Design review of the part built by this model. Coordinates are the model's own, in mm. Face numbers are marked on the shaded views. A direction names the side the tool comes from. Coordinates: 2 decimals unless noted, no trailing zeros. Loops run counter-clockwise (first coordinate to the right, second up) from the corner with the lowest first, then second, coordinate; pieces in that order, holes last.
Q1. Machinability: for the marked faces 4, 5 and 6, which of the approach directions +Z, -Z, +X, -X, +Y, -Y give a long, thin tool a straight path to every point of the face, cutting with its end or side? Answer none if there is none.
Q2. Wall thickness on probe 1 along Y at (x, z) = (0, 20); probe 2 along Y at (x, z) = (23.5, 9.5); probe 3 along Z at (x, y) = (8, 41): over which ranges is each line inside the solid? List them lowest first.
Q3. Add section A-A on x = 0. Give the boundary of the cut face in (y, z), and give its area (3 significant figures).
Q4. Add section C-C on x = -29.5. Give the boundary of the cut face in (y, z).
Q5. Draft analysis for pull direction X (two halves, no side actions). For the marked faces 1, 2 and 3, state which applies: released by +X, released by -X, zero draft, split by the parting line, or undercut.
Q6. Add section B-B on z = 30. Give the boundary of the cut face in (x, y).
Q7. For P1, Ø2, axis at x = -6.5, z = 31, coming from the -Y side; P2, Ø3, axis at x = 28.5, y = 12, coming from the +Z side; P3, Ø4, axis at x = -10.5, z = 16.5, coming from the +Y side; P4, Ø8, axis at y = 31, z = 22, coming from the +X side (3 decimals), all flat-tipped, find the tip position at first contact; note any pin that passes through.
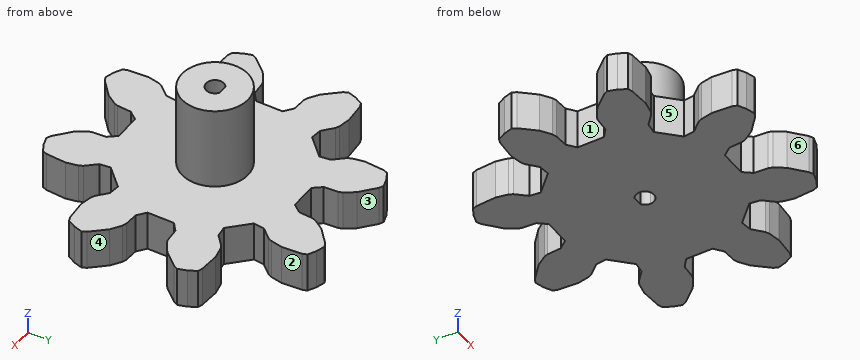
```python
from build123d import *

# Parameters (mm, degrees)
F1_DEPTH = 15.24
F2_R     = 12.7
F3_DEPTH = 31.75
F4_DEPTH = 25.4


with BuildPart() as f1:
    # F0 (on Top) → F1 (new body)
    with BuildSketch(Plane.XY):
        Polygon((-48.986719159, 25.3412460777), (-50.7255351294, 24.7465363945), (-52.3601977854, 21.688304154), (-53.366815822, 18.3699267661), (-52.5578082129, 16.719871907), (-47.6057296253, 11.0468524364), (-43.80914346, 8.4974130761), (-42.2801519731, 7.9744654227), (-37.0147232049, 7.6171909331), (-33.782, 5.0679251692), (-33.782, -5.0679251692), (-37.0147232049, -7.6171909331), (-42.2801519731, -7.9744654227), (-43.80914346, -8.4974130761), (-47.6057296253, -11.0468524364), (-52.5578082129, -16.719871907), (-53.366815822, -18.3699267661), (-52.3601977854, -21.688304154), (-50.7255351294, -24.7465363945), (-48.986719159, -25.3412460777), (-41.4736370284, -25.8510271212), (-36.9863201834, -24.9691669416), (-35.5353802528, -24.2577827562), (-31.559527, -20.7871925925), (-27.4710453735, -20.303918365), (-20.303918365, -27.4710453735), (-20.7871925925, -31.559527), (-24.2577827562, -35.5353802528), (-24.9691669416, -36.9863201834), (-25.8510271212, -41.4736370284), (-25.3412460777, -48.986719159), (-24.7465363945, -50.7255351294), (-21.688304154, -52.3601977854), (-18.3699267661, -53.366815822), (-16.719871907, -52.5578082129), (-11.0468524364, -47.6057296253), (-8.4974130761, -43.80914346), (-7.9744654227, -42.2801519731), (-7.6171909331, -37.0147232049), (-5.0679251692, -33.782), (5.0679251692, -33.782), (7.6171909331, -37.0147232049), (7.9744654227, -42.2801519731), (8.4974130761, -43.80914346), (11.0468524364, -47.6057296253), (16.719871907, -52.5578082129), (18.3699267661, -53.366815822), (21.688304154, -52.3601977854), (24.7465363945, -50.7255351294), (25.3412460777, -48.986719159), (25.8510271212, -41.4736370284), (24.9691669416, -36.9863201834), (24.2577827562, -35.5353802528), (20.7871925925, -31.559527), (20.303918365, -27.4710453735), (27.4710453735, -20.303918365), (31.559527, -20.7871925925), (35.5353802528, -24.2577827562), (36.9863201834, -24.9691669416), (41.4736370284, -25.8510271212), (48.986719159, -25.3412460777), (50.7255351294, -24.7465363945), (52.3601977854, -21.688304154), (53.366815822, -18.3699267661), (52.5578082129, -16.719871907), (47.6057296253, -11.0468524364), (43.80914346, -8.4974130761), (42.2801519731, -7.9744654227), (37.0147232049, -7.6171909331), (33.782, -5.0679251692), (33.782, 5.0679251692), (37.0147232049, 7.6171909331), (42.2801519731, 7.9744654227), (43.80914346, 8.4974130761), (47.6057296253, 11.0468524364), (52.5578082129, 16.719871907), (53.366815822, 18.3699267661), (52.3601977854, 21.688304154), (50.7255351294, 24.7465363945), (48.986719159, 25.3412460777), (41.4736370284, 25.8510271212), (36.9863201834, 24.9691669416), (35.5353802528, 24.2577827562), (31.559527, 20.7871925925), (27.4710453735, 20.303918365), (20.303918365, 27.4710453735), (20.7871925925, 31.559527), (24.2577827562, 35.5353802528), (24.9691669416, 36.9863201834), (25.8510271212, 41.4736370284), (25.3412460777, 48.986719159), (24.7465363945, 50.7255351294), (21.688304154, 52.3601977854), (18.3699267661, 53.366815822), (16.719871907, 52.5578082129), (11.0468524364, 47.6057296253), (8.4974130761, 43.80914346), (7.9744654227, 42.2801519731), (7.6171909331, 37.0147232049), (5.0679251692, 33.782), (-5.0679251692, 33.782), (-7.6171909331, 37.0147232049), (-7.9744654227, 42.2801519731), (-8.4974130761, 43.80914346), (-11.0468524364, 47.6057296253), (-16.719871907, 52.5578082129), (-18.3699267661, 53.366815822), (-21.688304154, 52.3601977854), (-24.7465363945, 50.7255351294), (-25.3412460777, 48.986719159), (-25.8510271212, 41.4736370284), (-24.9691669416, 36.9863201834), (-24.2577827562, 35.5353802528), (-20.7871925925, 31.559527), (-20.303918365, 27.4710453735), (-27.4710453735, 20.303918365), (-31.559527, 20.7871925925), (-35.5353802528, 24.2577827562), (-36.9863201834, 24.9691669416), (-41.4736370284, 25.8510271212), align=None)
        Polygon((-6.457554456, 6.1279886028), (-5.0423575535, 7.3366771559), (-3.4067913067, 8.2247200336), (-1.622328418, 8.7533028893), (0.2330374214, 8.8993240645), (2.0782189459, 8.6564005578), (3.8325695574, 8.0351529003), (5.4194220185, 7.0627288788), (6.7694179402, 5.7816284228), (7.8235568446, 4.247847459), (8.5357689507, 2.5284119549), (8.8749315621, 0.6984712932), (8.8262133252, -1.1619911548), (8.3917463583, -2.9716744665), (7.5905194232, -4.6514766054), (6.457554456, -6.1279886028), (5.0423575535, -7.3366771559), (3.4067913067, -8.2247200336), (1.622328418, -8.7533028893), (-0.2330374214, -8.8993240645), (-2.0782189459, -8.6564005578), (-3.8325695574, -8.0351529003), (-5.4194220185, -7.0627288788), (-6.7694179402, -5.7816284228), (-7.8235568446, -4.247847459), (-8.5357689507, -2.5284119549), (-8.8749315621, -0.6984712932), (-8.8262133252, 1.1619911548), (-8.3917463583, 2.9716744665), (-7.5905194232, 4.6514766054), align=None, mode=Mode.SUBTRACT)
        Polygon((-3.4067913067, 8.2247200336), (-5.0423575535, 7.3366771559), (-6.457554456, 6.1279886028), (-7.5905194232, 4.6514766054), (-8.3917463583, 2.9716744665), (-8.8262133252, 1.1619911548), (-8.8749315621, -0.6984712932), (-8.5357689507, -2.5284119549), (-7.8235568446, -4.247847459), (-6.7694179402, -5.7816284228), (-5.4194220185, -7.0627288788), (-3.8325695574, -8.0351529003), (-2.0782189459, -8.6564005578), (-0.2330374214, -8.8993240645), (1.622328418, -8.7533028893), (3.4067913067, -8.2247200336), (5.0423575535, -7.3366771559), (6.457554456, -6.1279886028), (7.5905194232, -4.6514766054), (8.3917463583, -2.9716744665), (8.8262133252, -1.1619911548), (8.8749315621, 0.6984712932), (8.5357689507, 2.5284119549), (7.8235568446, 4.247847459), (6.7694179402, 5.7816284228), (5.4194220185, 7.0627288788), (3.8325695574, 8.0351529003), (2.0782189459, 8.6564005578), (0.2330374214, 8.8993240645), (-1.622328418, 8.7533028893), align=None)
    extrude(amount=F1_DEPTH)

    # F2 (on face) → F3 (join)
    with BuildSketch(Plane.XY.offset(15.24)):
        Circle(F2_R)
        with BuildLine():
            ThreePointArc((1.7960512242, 2.921), (2.9930503377, 1.6732276223), (3.429, 0))
            ThreePointArc((3.429, 0), (-1.6732276223, -2.9930503377), (-1.7960512242, 2.921))
            ThreePointArc((-1.7960512242, 2.921), (0, 3.429), (1.7960512242, 2.921))
        make_face(mode=Mode.SUBTRACT)
        with BuildLine():
            Line((-1.7960512242, 2.921), (1.7960512242, 2.921))
            ThreePointArc((1.7960512242, 2.921), (0, 3.429), (-1.7960512242, 2.921))
        make_face()
    extrude(amount=F3_DEPTH)

    # F4 (cut): a face of the model
    f4_faces = [f1.faces().sort_by_distance(p)[0] for p in [
        (0, -0.108182678, 15.24),
    ]]
    extrude(f4_faces, amount=-F4_DEPTH, mode=Mode.SUBTRACT)


solid = f1.part
```
Entries:
1. face 4: +Z, -Z, +X
1. face 5: +Z, -Z
1. face 6: +Z, -Z, -Y
2. probe 1: y = -12.7 to -3.43, 2.92 to 12.7
2. probe 2: y = -51.39 to -34.67, -24.27 to 24.27, 34.67 to 51.39
2. probe 3: z = 0 to 15.24
3. outline: (-33.78, 0) - (-3.43, 0) - (-3.43, 46.99) - (-12.7, 46.99) - (-12.7, 15.24) - (-33.78, 15.24) - close; (2.92, 0) - (33.78, 0) - (33.78, 15.24) - (12.7, 15.24) - (12.7, 46.99) - (2.92, 46.99) - close
3. area: 1,540 mm2
4. outline: (-20.54, 0) - (20.54, 0) - (20.54, 15.24) - (-20.54, 15.24) - close
5. face 1: released by -X
5. face 2: released by +X
5. face 3: undercut
6. outline: circle Ø25.4 at (0, 0); hole (-1.8, 2.92) arc R3.43 ccw (long way) to (1.8, 2.92) - close
7. P1: stops at y = -11.45
7. P2: stops at z = 15.24
7. P3: stops at y = 48.48
7. P4: passes through
